```python
from build123d import *

# Parameters (mm, degrees)
BOSS_EXTRUDE1_DEPTH = 22
SKETCH2_W           = 68
SKETCH2_H           = 3
BOSS_EXTRUDE2_DEPTH = 22
BOSS_EXTRUDE3_DEPTH = 14
CUT_EXTRUDE1_DEPTH  = 10
SKETCH5_R           = 1.15
SKETCH5_W           = 3
SKETCH5_H           = 74
CUT_EXTRUDE2_DEPTH  = 1.5


with BuildPart() as part:
    # Sketch1 → Boss-Extrude1 (new body)
    with BuildSketch(Plane(origin=(0, 0, 0), x_dir=(1, 0, 0), z_dir=(0, 1, 0))):
        Polygon((14, 14), (11.5, 14), (11.5, 34), (9, 34), (9, -34), (11.5, -34), (11.5, -14), (14, -14), align=None)
    extrude(amount=BOSS_EXTRUDE1_DEPTH)

    # Sketch2 → Boss-Extrude2 (add)
    with BuildSketch(Plane.ZY.offset(-9)):
        with Locations((0, 20.5)):
            Rectangle(SKETCH2_W, SKETCH2_H)
    extrude(amount=BOSS_EXTRUDE2_DEPTH)

    # Sketch3 → Boss-Extrude3 (add)
    with BuildSketch(Plane(origin=(0, 22, 0), x_dir=(1, 0, 0), z_dir=(0, 1, 0))):
        Polygon((-13, 34), (11.5, 34), (11.5, 37), (-16, 37), (-16, -37), (11.5, -37), (11.5, -34), (-13, -34), align=None)
    extrude(amount=-BOSS_EXTRUDE3_DEPTH)

    # Sketch4 → Cut-Extrude1 (cut)
    with BuildSketch(Plane.XY.offset(37)):
        Polygon((7, 13.5), (-11, 13.5), (-13, 13.5), (-13, 8), (-11, 8), (7, 8), (9, 8), (9, 13.5), align=None)
    extrude(amount=-CUT_EXTRUDE1_DEPTH, mode=Mode.SUBTRACT)

    # Sketch5 → Cut-Extrude2 (cut)
    with BuildSketch(Plane(origin=(0, 22, 0), x_dir=(1, 0, 0), z_dir=(0, 1, 0))):
        with Locations(Location((9, 34, 0), (0, 0, 270))):
            Circle(SKETCH5_R)
        with Locations(Location((9, -34, 0), (0, 0, 270))):
            Circle(SKETCH5_R)
        with Locations(Location((-13, -34, 0), (0, 0, 270))):
            Circle(SKETCH5_R)
        with Locations(Location((-13, 34, 0), (0, 0, 270))):
            Circle(SKETCH5_R)
        with Locations((-7.5, 0)):
            Rectangle(SKETCH5_W, SKETCH5_H)
    extrude(amount=-CUT_EXTRUDE2_DEPTH, mode=Mode.SUBTRACT)


solid = part.part
```
Check sheet for the modelled part. Datum: model origin and axes. Units: mm. A direction names the side the tool comes from. Round coordinates to 2 decimals unless told otherwise and drop trailing zeros. Order: outer loops, then holes, each group sorted by start corner. A loop starts at its lowest first (then second) coordinate and runs counter-clockwise, first axis right, second up. Notation, with made-up numbers: M -12.75,71 L 27.25,71 A34 cw 27.25,108 Z; hole C -8,-29.5 d6. An arc over 180 degrees is marked long. Answer in a Markdown table with one row per item.
(1) Section check A-A on y = 17.25. Record the boundary of the cut face in (x, z).
Findings:
| item | result |
|---|---|
| outline | M -16,-37 L 11.5,-37 L 11.5,-14 L 14,-14 L 14,14 L 11.5,14 L 11.5,37 L -16,37 Z; hole M -13,-34 L 9,-34 L 9,34 L -13,34 Z |
(2) Material ranges on line 1 along X through (y, z) = (20.85, -34); line 2 along X through (y, z) = (14.75, 7); line 3 along X through (y, z) = (15.5, -18), recorded low to high. Write a range as from..to.
Findings:
| item | result |
|---|---|
| line 1 | x = -16..-14.15, -11.85..-9, -6..7.85, 10.15..11.5 |
| line 2 | x = -16..-13, 9..14 |
| line 3 | x = -16..-13, 9..11.5 |
(3) Section check D-D on y = 6.5. Record the boundary of the cut face in (x, z), plus the area to 3 significant figures.
Findings:
| item | result |
|---|---|
| outline | M 9,-34 L 11.5,-34 L 11.5,-14 L 14,-14 L 14,14 L 11.5,14 L 11.5,34 L 9,34 Z |
| area | 240 mm^2 |
(4) Section check C-C on z = 13. Record the boundary of the cut face in (x, y), plus the area to 4 significant figures.
Findings:
| item | result |
|---|---|
| outline | M -16,8 L -13,8 L -13,19 L 9,19 L 9,0 L 14,0 L 14,22 L -6,22 L -6,20.5 L -9,20.5 L -9,22 L -16,22 Z |
| area | 213.5 mm^2 |
(5) Gauge pin test, flat ends, axial feed: pin 1 (2 mm diameter, centred on x = 9, z = -34, fed in from +Y); pin 2 (0.8 mm diameter, centred on x = 11, z = 35.5, fed in from -Y); pin 3 (0.9 mm diameter, centred on x = -3, z = 35, fed in from -Y). Record the tip position at first contact, or that the pin passes through.
Findings:
| item | result |
|---|---|
| pin 1 | stops at y = 20.5 |
| pin 2 | stops at y = 8 |
| pin 3 | stops at y = 13.5 |
(6) Section check B-B on x = 1. Record the boundary of the cut face in (y, z).
Findings:
| item | result |
|---|---|
| outline | M 8,-37 L 22,-37 L 22,37 L 13.5,37 L 13.5,34 L 19,34 L 19,-34 L 8,-34 Z |
(7) Set-up check for faces 1 (the cylindrical face through (8.56, 21.26, 35.062)), 2 (the flat face through (-8, 20.5, -1)), 3 (the flat face through (13, 11, -14)), 4 (the flat face through (11.5, 11, 26)), 5 (the flat face through (-2, 16, 34)): record each of +Z, -Z, +X, -X, +Y, -Y from which the full face is reachable in a straight line by a thin tool's end or side.
Findings:
| item | result |
|---|---|
| face 1 | +Y |
| face 2 | +Z, -Z, +Y |
| face 3 | -Z, +X, +Y, -Y |
| face 4 | +Z, +X, +Y, -Y |
| face 5 | -Y |
